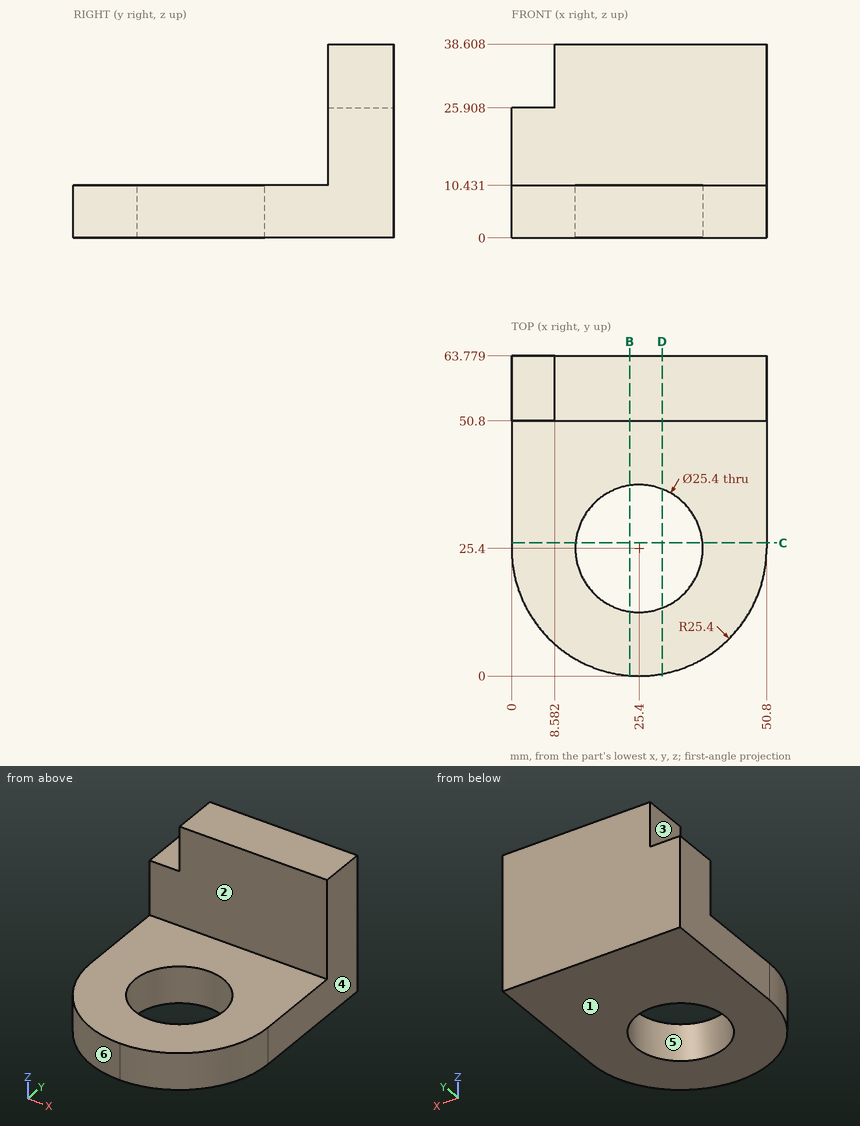
The drawing under review shows one solid part. Ordinate dimensions are in mm from its lowest x, y, z. A direction names the side the tool comes from. Round coordinates to 2 decimals unless told otherwise and drop trailing zeros. Order: outer loops, then holes, each group sorted by start corner. A loop starts at its lowest first (then second) coordinate and runs counter-clockwise, first axis right, second up. Notation, with made-up numbers: (-37, 30) -> (-3, 30) arc R16 ccw to (-3, 35) -> close; hole circle Ø7 at (-7.75, -28). An arc over 180 degrees is marked (long way). Use a Markdown table: item, result.
Q1. We need section B-B on x = 23.5. Write out the cut boundary in (y, z), then the cut area to 3 significant figures.
Values:
| item | result |
|---|---|
| outline | (0.07, 0) -> (12.84, 0) -> (12.84, 10.43) -> (0.07, 10.43) -> close; (37.96, 0) -> (63.78, 0) -> (63.78, 38.61) -> (50.8, 38.61) -> (50.8, 10.43) -> (37.96, 10.43) -> close |
| area | 768 mm^2 |
Q2. Clearance check with flat-ended pins moving along their axes: P1, Ø10, axis at y = 57.5, z = 33, coming from the -X side; P2, Ø10, axis at y = 14.5, z = 10, coming from the +X side (1 decimal); P3, Ø9.5, axis at x = 4, y = 56, coming from the +Z side; P4, Ø2, axis at x = 9, z = 5, coming from the -Y side. State where each tip first meets the part, or that it passes through.
Values:
| item | result |
|---|---|
| P1 | stops at x = 8.58 |
| P2 | stops at x = 50.1 |
| P3 | stops at z = 38.61 |
| P4 | stops at y = 5.2 |
Q3. We need section C-C on y = 26.5. Write out the cut boundary in (x, z).
Values:
| item | result |
|---|---|
| outline | (0, 0) -> (12.75, 0) -> (12.75, 10.43) -> (0, 10.43) -> close; (38.05, 0) -> (50.8, 0) -> (50.8, 10.43) -> (38.05, 10.43) -> close |
Q4. We need section D-D on x = 30. Write out the cut boundary in (y, z).
Values:
| item | result |
|---|---|
| outline | (0.42, 0) -> (13.56, 0) -> (13.56, 10.43) -> (0.42, 10.43) -> close; (37.24, 0) -> (63.78, 0) -> (63.78, 38.61) -> (50.8, 38.61) -> (50.8, 10.43) -> (37.24, 10.43) -> close |
Q5. For line 1 (Y direction, x = 25, z = 2); line 2 (X direction, y = 25, z = 4); line 3 (Y direction, x = 18.5, z = 31), list the stretches that pass through material, from the lowest coordinate up.
Values:
| item | result |
|---|---|
| line 1 | y = 0 to 12.71, 38.09 to 63.78 |
| line 2 | x = 0 to 12.71, 38.09 to 50.8 |
| line 3 | y = 50.8 to 63.78 |
Q6. Tool access review of the marked faces 1, 2 and 3: name each direction out of +Z, -Z, +X, -X, +Y, -Y from which nothing blocks a thin tool from reaching the whole face with its end or side.
Values:
| item | result |
|---|---|
| face 1 | -Z, +X, -X, +Y, -Y |
| face 2 | +Z, +X, -X, -Y |
| face 3 | +Z, -X, +Y, -Y |
Q7. Mouldability with a two-part tool opening along X and no side actions: class the marked faces 4, 5 and 6 as +X half, -X half, draft (parallel to the pull), parting line (faces both ways), or undercut.
Values:
| item | result |
|---|---|
| face 4 | +X half |
| face 5 | undercut |
| face 6 | -X half |
